Design review of the part built by this model. Coordinates are the model's own, in mm. A direction names the side the tool comes from. Coordinates: 2 decimals unless noted, no trailing zeros. Loops run counter-clockwise (first coordinate to the right, second up) from the corner with the lowest first, then second, coordinate; pieces in that order, holes last.
Q1. Machinability: for faces 1 (the face through (62, -12.7, 0)), 2 (the face through (52, -10.2, 0)), which of the approach directions +Z, -Z, +X, -X, +Y, -Y give a long, thin tool a straight path to every point of the face, cutting with its end or side? Answer none if there is none.
Q2. Draft analysis for pull direction Z (two halves, no side actions). For faces 3 (the face through (12.5, -11.1, -0.2)), 4 (the face through (102.7, 0, -11)), 5 (the face through (52, 0, -10.2)), state which applies: released by +Z, released by -Z, zero draft, split by the parting line, or undercut.
Q3. For P1, Ø10, axis at y = -4, z = 6.5, coming from the +X side, flat-tipped, find the tip position at first contact; note if it passes through.
Q4. Add section A-A on z = 0.5. Give the boundary of the cut face in (x, y), and give its area (4 significant figures).
Q5. Add section D-D on x = 76. Give the boundary of the cut face in (y, z), and give its area (3 significant figures).
Q6. Add section C-C on x = 12. Give the boundary of the cut face in (y, z), and give its area (3 significant figures).
Q7. Wall thickness on probe 1 along Z at (x, y) = (92.5, 5.25); probe 2 along Z at (x, y) = (12, 0.75): over which ranges is each line inside the solid? List them lowest first.
Q8. Add section B-B on y = -8.5. Give the boundary of the cut face in (x, z), and give its area (3 significant figures).
```python
from build123d import *

# Parameters (mm, degrees)
SKETCH2_W           = 25.4
SKETCH2_H           = 25.4
SKETCH2_W_2         = 20.4
SKETCH2_H_2         = 20.4
BOSS_EXTRUDE1_DEPTH = 102.7
CUT_EXTRUDE1_DEPTH  = 107.553930007


with BuildPart() as part:
    # Sketch2 → Boss-Extrude1 (new body)
    with BuildSketch(Plane(origin=(0, 0, 0), x_dir=(0, 0, -1), z_dir=(1, 0, 0))):
        Rectangle(SKETCH2_W, SKETCH2_H)
        Rectangle(SKETCH2_W_2, SKETCH2_H_2, mode=Mode.SUBTRACT)
    extrude(amount=BOSS_EXTRUDE1_DEPTH)

    # Sketch3 → Cut-Extrude1 (cut, through all)
    with BuildSketch(Plane(origin=(0, 12.7, 0), x_dir=(1, 0, 0), z_dir=(0, 1, 0))):
        Polygon((0, -12.7), (0, 12.7), (25.4, -12.7), align=None)
    extrude(amount=-CUT_EXTRUDE1_DEPTH, mode=Mode.SUBTRACT)


solid = part.part
```
Entries:
1. face 1: +Z, -Z, +X, -X, -Y
1. face 2: +X, -X
2. face 3: released by +Z
2. face 4: zero draft
2. face 5: undercut
3. P1: stops at x = 102.7
4. outline: (13.2, -12.7) - (102.7, -12.7) - (102.7, -10.2) - (13.2, -10.2) - close; (13.2, 10.2) - (102.7, 10.2) - (102.7, 12.7) - (13.2, 12.7) - close
4. area: 447.5 mm2
5. outline: (-12.7, -12.7) - (12.7, -12.7) - (12.7, 12.7) - (-12.7, 12.7) - close; hole (-10.2, -10.2) - (10.2, -10.2) - (10.2, 10.2) - (-10.2, 10.2) - close
5. area: 229 mm2
6. outline: (-12.7, -12.7) - (12.7, -12.7) - (12.7, -0.7) - (10.2, -0.7) - (10.2, -10.2) - (-10.2, -10.2) - (-10.2, -0.7) - (-12.7, -0.7) - close
6. area: 111 mm2
7. probe 1: z = -12.7 to -10.2, 10.2 to 12.7
7. probe 2: z = -12.7 to -10.2
8. outline: (0, -12.7) - (102.7, -12.7) - (102.7, -10.2) - (2.5, -10.2) - close; (22.9, 10.2) - (102.7, 10.2) - (102.7, 12.7) - (25.4, 12.7) - close
8. area: 450 mm2
